CAD build for the part. Positions are in the model's coordinates, mm. Round coordinates to 2 decimals unless told otherwise and drop trailing zeros. Loops run counter-clockwise (first coordinate to the right, second up) from the corner with the lowest first, then second, coordinate; pieces in that order, holes last. Notation, with made-up numbers: (-20.75, 77) - (13.25, 77) arc R26 cw to (13.25, 112) - close; hole circle Ø7 at (51.25, 1.25). An arc over 180 degrees is marked (long way). One line per question, with ' | ' between items.
```python
from build123d import *

# Parameters (mm, degrees)
EXTRUDE1_DEPTH = 0.16
SKETCH2_R      = 0.05
EXTRUDE2_DEPTH = 1.32


with BuildPart() as part:
    # Sketch1 → Extrude1 (new body, symmetric)
    with BuildSketch(Plane(origin=(0, 0, 0), x_dir=(-1, 0, 0), z_dir=(0, 0, -1))):
        Polygon((-4.387, 43.998003308), (4.387, 43.998003308), (12.697, 170.784102838), (-12.697, 170.784102838), align=None)
    extrude(amount=EXTRUDE1_DEPTH, both=True)

    # Sketch2 → Extrude2 (cut, through all)
    with BuildSketch(Plane.XY.offset(0.16)):
        with Locations((-3, 44.198003308)):
            Circle(SKETCH2_R)
        with Locations((0, 44.198003308)):
            Circle(SKETCH2_R)
        with Locations(Location((3, 44.198003308, 0), (0, 0, 180))):  # turned: the seam where the file's is
            Circle(SKETCH2_R)
        with Locations((0, 170.583003308)):
            Circle(SKETCH2_R)
        with Locations((-10, 170.583003308)):
            Circle(SKETCH2_R)
        with Locations(Location((10, 170.583003308, 0), (0, 0, 180))):  # turned: the seam where the file's is
            Circle(SKETCH2_R)
    extrude(amount=-EXTRUDE2_DEPTH, mode=Mode.SUBTRACT)


solid = part.part
```
(1) Cut at C-C, the plane x = 5.5. Write the cut outline in (y, z), then the cut area to 3 significant figures.
Results found:
outline: (60.98, -0.16) - (170.78, -0.16) - (170.78, 0.16) - (60.98, 0.16) - close | area: 35.1 mm²
(2) Cut at A-A, the plane z = 0. Write the cut outline in (x, y).
Results found:
outline: (-12.7, 170.78) - (-4.39, 44) - (4.39, 44) - (12.7, 170.78) - close; hole circle Ø0.1 at (-10, 170.58); hole circle Ø0.1 at (-3, 44.2); hole circle Ø0.1 at (0, 44.2); hole circle Ø0.1 at (0, 170.58); hole circle Ø0.1 at (3, 44.2); hole circle Ø0.1 at (10, 170.58)
(3) Probe L1, parallel to X at y = 92, z = 0; L2, parallel to X at y = 88.5, z = 0.1. List the from-to ranges inside material, lowest first.
Results found:
L1: x = -7.53 to 7.53 | L2: x = -7.3 to 7.3
(4) Cut at B-B, the plane y = 141.5. Write the cut outline in (x, z), then the cut area to 3 significant figures.
Results found:
outline: (-10.78, -0.16) - (10.78, -0.16) - (10.78, 0.16) - (-10.78, 0.16) - close | area: 6.90 mm²
